Can you work these out from the model? Positions are in its coordinate system, mm. A direction names the side the tool comes from. Give positions to 0.01 mm unless a question says otherwise; leave off trailing zeros. Write each loop counter-clockwise with the first axis right and the second up, starting at its lowest first coordinate (ties: lowest second). Pieces come first, ordered by that corner, then holes.
from build123d import *

# Parameters (mm, degrees)
F0_R     = 15.24
F1_DEPTH = 31.75
F2_R     = 3.81
F3_R     = 2.413
F4_DEPTH = 152.4


with BuildPart() as f1:
    # F0 (on Front) → F1 (new body)
    with BuildSketch(Plane.XZ):
        Circle(F0_R)
    extrude(amount=F1_DEPTH)

    # F2
    f2_edges = [f1.edges().sort_by_distance(p)[0] for p in [
        (-15.24, -31.75, 0),
        (-15.24, 0, 0),
    ]]
    fillet(f2_edges, radius=F2_R)

    # F3 (on face) → F4 (join)
    with BuildSketch(Plane(origin=(0, 0, 0), x_dir=(-1, 0, 0), z_dir=(0, 1, 0))):
        Circle(F3_R)
    extrude(amount=F4_DEPTH)


solid = f1.part
(1) For faces 3 (the face through (0, 152.4, 0)), 4 (the face through (1.915, 75.133, -1.468)), which set-ups out of +Z, -Z, +X, -X, +Y, -Y let a thin tool reach every point of the face, with its end or its side?
Returned:
face 3: +Z, -Z, +X, -X, +Y
face 4: +Y
(2) Imagine slicing it at B-B, the plane z = 0. Write out the boundary of the cut face in (x, y).
Returned:
outline: (-15.24, -27.94) arc R3.81 ccw to (-11.43, -31.75) - (11.43, -31.75) arc R3.81 ccw to (15.24, -27.94) - (15.24, -3.81) arc R3.81 ccw to (11.43, 0) - (2.41, 0) - (2.41, 152.4) - (-2.41, 152.4) - (-2.41, 0) - (-11.43, 0) arc R3.81 ccw to (-15.24, -3.81) - close
(3) Imagine slicing it at A-A, the plane x = 0. Write out the boundary of the cut face in (y, z), plus the area to 3 significant figures.
Returned:
outline: (-31.75, -11.43) arc R3.81 ccw to (-27.94, -15.24) - (-3.81, -15.24) arc R3.81 ccw to (0, -11.43) - (0, -2.41) - (152.4, -2.41) - (152.4, 2.41) - (0, 2.41) - (0, 11.43) arc R3.81 ccw to (-3.81, 15.24) - (-27.94, 15.24) arc R3.81 ccw to (-31.75, 11.43) - close
area: 1,690 mm2
(4) Imagine slicing it at C-C, the plane y = 37.5. Write out the boundary of the cut face in (x, z).
Returned:
outline: circle Ø4.83 at (0, 0)
(5) Will these pins go through, and if not, where does the flat tip stop? P1, Ø2, axis at x = 0, y = 2.5, coming from the +Z side; P2, Ø6, axis at x = -9, z = 1.5, coming from the +Y side; P3, Ø3, axis at x = -3.5, y = 46.5, coming from the +Z side.
Returned:
P1: stops at z = 2.41
P2: stops at y = 0
P3: stops at z = 1.35
(6) If I drill on L1, parallel to Y at x = 1, z = -7.5; L2, parallel to Z at x = 0, y = 4.5; L3, parallel to Y at x = -10.5, z = -5, over which ranges is the centre line in solid material (lowest first)?
Returned:
L1: y = -31.75 to 0
L2: z = -2.41 to 2.41
L3: y = -31.74 to -0.01
(7) Imagine slicing it at D-D, the plane y = -15.5. Write out the boundary of the cut face in (x, z).
Returned:
outline: circle Ø30.48 at (0, 0)
(8) If we mould it in two halves opening along X, with no side actions, what happens to faces 1 (the face through (-3.3, -15.71, -14.88)), 2 (the face through (0, -31.75, 0))? For each: +X half, -X half, draft (parallel to the pull), parting line (faces both ways), or undercut.
Returned:
face 1: parting line
face 2: draft
